```python
from build123d import *

# Parameters (mm, degrees)
F2_R = 6.34999


# Not quite as in the source:
# - a fillet or chamfer is up to 0.001 mm smaller than in the source, because OpenCascade refuses the exact size


with BuildPart() as f1:
    # F0 (on Front) → F1 (revolve)
    with BuildSketch(Plane.XZ):
        Polygon((3.9624, -5.7219677535), (0, -5.7219677535), (0, -23.1971677535), (113.5126, -23.1971677535), (113.5126, -16.8471677535), (3.9624, -16.8471677535), align=None)
    revolve(axis=Axis((1.9812, 0, -3.3343677535), (1, 0, 0)))

    # F2 (radius 6.35 in the source; OpenCascade refuses exactly that, so slightly less here)
    f2_edges = [f1.edges().sort_by_distance(p)[0] for p in [
        (0, 0, 16.528432),
        (113.5126, 0, 16.528432),
    ]]
    fillet(f2_edges, radius=F2_R)


solid = f1.part
```
Can you work these out from the model? Positions are in its coordinate system, mm. A direction names the side the tool comes from. Round coordinates to 2 decimals unless told otherwise and drop trailing zeros. Loops run counter-clockwise (first coordinate to the right, second up) from the corner with the lowest first, then second, coordinate; pieces in that order, holes last. Notation, with made-up numbers: (31, 72) -> (75, 72) arc R11 ccw to (75, 81) -> close; hole circle Ø6 at (51, 29). An arc over 180 degrees is marked (long way). One line per item, written item: value. Start each with the question number.
1. For faces 1 (the cylindrical face through (1.95, 0.1, -0.95)), 2 (the flat face through (3.962, 0, -6)), which set-ups out of +Z, -Z, +X, -X, +Y, -Y let a thin tool reach every point of the face, with its end or its side?
2. For pin 1 (1.5 mm diameter, centred on x = 67.5, z = 3.5, fed in from -Y); pin 2 (2 mm diameter, centred on y = -11.5, z = -13, fed in from -X); pin 3 (2 mm diameter, centred on x = 91.5, z = 2.5, fed in from -Y); pin 4 (4 mm diameter, centred on y = 0, z = -3.33, fed in from -X), each with a flat end and sliding along its axis, tell me the tip position at first contact or that it passes through.
3. If we section it at B-B, the plane x = 69: Write out the boundary of the cut face in (y, z).
4. If I drill on probe 1 along X at (y, z) = (-12, -1); probe 2 along Y at (x, z) = (48.5, -2); probe 3 along X at (y, z) = (-3, -17), over which ranges is the centre line in solid material (lowest first)?
5. If we mould it in two halves opening along Z, with no side actions, what happens to faces 3 (the flat face through (0, 0.2, -0.5)), 4 (the cylindrical face through (57.462, -12.086, 12.428)), 5 (the cylindrical face through (57.971, 4.059, -16.223))? For each: pulls with the +Z half, pulls with the -Z half, needs draft (parallel to the pull), parting line crosses it, or undercut.
Calculated:
1. face 1: +X, -X
1. face 2: +X
2. pin 1: stops at y = -18.91
2. pin 2: stops at x = 0.02
2. pin 3: stops at y = -19.27
2. pin 4: passes through
3. outline: circle Ø39.73 at (0, -3.33); hole circle Ø27.03 at (0, -3.33)
4. probe 1: x = 0 to 3.96
4. probe 2: y = -19.82 to -13.45, 13.45 to 19.82
4. probe 3: x = 0.02 to 113.49
5. face 3: needs draft
5. face 4: parting line crosses it
5. face 5: undercut
